Source: CAD feature listing. Evaluate the final solid. Frame: model axes, mm. A direction names the side the tool comes from. Give positions to 0.01 mm unless a question says otherwise; leave off trailing zeros. Order: outer loops, then holes, each group sorted by start corner. A loop starts at its lowest first (then second) coordinate and runs counter-clockwise, first axis right, second up. Notation, with made-up numbers: (26, 71.25) -> (67, 71.25) arc R11 cw to (67, 77.25) -> close; hole circle Ø8 at (86.5, -23). An arc over 180 degrees is marked (long way). Use CSV: the item, a comma, the result in double quotes.
```python
from build123d import *

# Parameters (mm, degrees)
SKETCH1_W           = 12
SKETCH1_H           = 16
BOSS_EXTRUDE1_DEPTH = 159.3
SKETCH2_W           = 14.8
SKETCH2_H           = 20
BOSS_EXTRUDE2_DEPTH = 37.4
SKETCH3_W           = 7.8
SKETCH3_H           = 4.5
BOSS_EXTRUDE3_DEPTH = 7.8
SKETCH4_R           = 2
CUT_EXTRUDE1_DEPTH  = 206.055943586
SKETCH5_W           = 6.1
SKETCH5_H           = 9
CUT_EXTRUDE2_DEPTH  = 192.2


with BuildPart() as part:
    # Sketch1 → Boss-Extrude1 (new body)
    with BuildSketch(Plane.XY):
        Rectangle(SKETCH1_W, SKETCH1_H)
    extrude(amount=BOSS_EXTRUDE1_DEPTH)

    # Sketch2 → Boss-Extrude2 (add)
    with BuildSketch(Plane.XY.offset(159.3)):
        Rectangle(SKETCH2_W, SKETCH2_H)
    extrude(amount=BOSS_EXTRUDE2_DEPTH)

    # Sketch3 → Boss-Extrude3 (add)
    with BuildSketch(Plane.XY.offset(196.7)):
        Rectangle(SKETCH3_W, SKETCH3_H)
    extrude(amount=BOSS_EXTRUDE3_DEPTH)

    # Sketch4 → Cut-Extrude1 (cut, through all)
    with BuildSketch(Plane.ZY.offset(3.9)):
        with Locations((200, 0)):
            Circle(SKETCH4_R)
        with BuildLine():
            Line((202.25, -2.25), (204.5, -2.25))
            Line((204.5, -2.25), (204.5, -3.3e-08))
            ThreePointArc((204.5, -3.3e-08), (203.840990246, -1.590990269), (202.25, -2.25))
        make_face()
        with BuildLine():
            ThreePointArc((202.25, 2.25), (203.840990269, 1.590990246), (204.5, -3.3e-08))
            Line((204.5, -3.3e-08), (204.5, 2.25))
            Line((204.5, 2.25), (202.25, 2.25))
        make_face()
    extrude(amount=-CUT_EXTRUDE1_DEPTH, mode=Mode.SUBTRACT)

    # Sketch5 → Cut-Extrude2 (cut)
    with BuildSketch(Plane(origin=(0, 0, 0), x_dir=(-1, 0, 0), z_dir=(0, 0, -1))):
        Rectangle(SKETCH5_W, SKETCH5_H)
    extrude(amount=-CUT_EXTRUDE2_DEPTH, mode=Mode.SUBTRACT)


solid = part.part
```
1. Pin query (flat end, axial travel): P1, Ø4, axis at x = 3.5, z = 54.5, coming from the -Y side; P2, Ø10, axis at y = 1, z = 59, coming from the -X side; P3, Ø5, axis at y = -1, z = 201.5, coming from the +X side; P4, Ø2, axis at x = 4.5, y = 5.5, coming from the -Z side. Return the tip coordinate at first contact, or that it passes through.
Answer below:
P1,"stops at y = -8"
P2,"stops at x = -6"
P3,"stops at x = 3.9"
P4,"stops at z = 0"
2. Ray query, line 1 along Y through (x, z) = (-1.5, 119.5); line 2 along X through (y, z) = (-4.25, 118); line 3 along Y through (x, z) = (1.5, 200). Return the intervals inside material, ascending.
Answer below:
line 1,"y = -8 to -4.5, 4.5 to 8"
line 2,"x = -6 to -3.05, 3.05 to 6"
line 3,"y = -2.25 to -2, 2 to 2.25"
3. Access query for faces 5 (the flat face through (-6, 0, 79)), 6 (the flat face through (0, 8, 79)), 7 (the flat face through (3.9, -2, 201)), 8 (the flat face through (6, 0, 79)). Directions: +Z, -Z, +X, -X, +Y, -Y. A direction counts if a zero-diameter tool reaches every point of the face in a straight line with its end or side. Return the directions, or none.
Answer below:
face 5,"-Z, -X, +Y, -Y"
face 6,"-Z, +X, -X, +Y"
face 7,"+Z, +X, +Y, -Y"
face 8,"-Z, +X, +Y, -Y"
4. Mould query, pull axis Y, two halves, no side actions, for faces 1 (the flat face through (0, 0, 192.2)), 2 (the flat face through (0, 4.5, 95)), 3 (the flat face through (7.4, 0, 178)), 4 (the flat face through (0, -2.25, 199)). Classes: released by +Y, released by -Y, zero draft, split by the parting line, or undercut.
Answer below:
face 1,"undercut"
face 2,"undercut"
face 3,"zero draft"
face 4,"released by -Y"
5. Section query B-B on z = 92. Return loops of the section in (x, y).
Answer below:
outline,"(-6, -8) -> (6, -8) -> (6, 8) -> (-6, 8) -> close; hole (-3.05, -4.5) -> (3.05, -4.5) -> (3.05, 4.5) -> (-3.05, 4.5) -> close"
6. Section query A-A on z = 185.5. Return loops of the section in (x, y).
Answer below:
outline,"(-7.4, -10) -> (7.4, -10) -> (7.4, 10) -> (-7.4, 10) -> close; hole (-3.05, -4.5) -> (3.05, -4.5) -> (3.05, 4.5) -> (-3.05, 4.5) -> close"
